from build123d import *

# Parameters (mm, degrees)
SKETCH1_R           = 5
BOSS_EXTRUDE1_DEPTH = 10
CUT_EXTRUDE2_DEPTH  = 10
FILLET1_R           = 2


with BuildPart() as part:
    # Sketch1 → Boss-Extrude1 (new body)
    # profile 1 of 2: a face of its own
    with BuildSketch(Plane.XY):
        with BuildLine():
            Line((0, 0), (0, 100))
            ThreePointArc((0, 100), (25, 125), (50, 100))
            Line((50, 100), (50, 0))
            ThreePointArc((50, 0), (25, -25), (0, 0))
        make_face()
        with BuildLine():
            ThreePointArc((15, 0), (25, -10), (35, 0))
            Line((35, 0), (35, 100))
            ThreePointArc((35, 100), (25, 110), (15, 100))
            Line((15, 100), (15, 0))
        make_face(mode=Mode.SUBTRACT)
    # profile 2 of 2: a face of its own
    with BuildSketch(Plane.XY):
        with BuildLine():
            Line((15, 0), (15, 100))
            ThreePointArc((15, 100), (25, 110), (35, 100))
            Line((35, 100), (35, 0))
            ThreePointArc((35, 0), (25, -10), (15, 0))
        make_face()
        with Locations((25, 0)):
            Circle(SKETCH1_R, mode=Mode.SUBTRACT)
        with Locations((25, 100)):
            Circle(SKETCH1_R, mode=Mode.SUBTRACT)
    extrude(amount=BOSS_EXTRUDE1_DEPTH)

    # Sketch2 → Cut-Extrude2 (cut)
    with BuildSketch(Plane.XY.offset(10)):
        with BuildLine():
            Line((25.064971157, 89.343145751), (10, 89.343145751))
            Line((10, 89.343145751), (10, 70.656854249))
            Line((10, 70.656854249), (26.125631329, 86.782485579))
            ThreePointArc((26.125631329, 86.782485579), (26.450790456, 88.417170899), (25.064971157, 89.343145751))
        make_face()
        with BuildLine():
            Line((40, 69), (40, 89.343145751))
            Line((40, 89.343145751), (22.217514421, 71.560660172))
            ThreePointArc((22.217514421, 71.560660172), (21.892355294, 69.925974851), (23.278174593, 69))
            Line((23.278174593, 69), (40, 69))
        make_face()
        with BuildLine():
            Line((26.721825407, 61), (10, 61))
            Line((10, 61), (10, 40.65685425))
            Line((10, 40.65685425), (22.171572875, 52.828427125))
            Line((22.171572875, 52.828427125), (27.782485579, 58.439339828))
            ThreePointArc((27.782485579, 58.439339828), (28.107644706, 60.074025149), (26.721825407, 61))
        make_face()
        with BuildLine():
            Line((40, 39), (40, 59.343145751))
            Line((40, 59.343145751), (27.828427125, 47.171572875))
            Line((27.828427125, 47.171572875), (22.217514421, 41.560660172))
            ThreePointArc((22.217514421, 41.560660172), (21.892355294, 39.925974852), (23.278174593, 39))
            Line((23.278174593, 39), (40, 39))
        make_face()
        with BuildLine():
            Line((26.721825408, 31.000000001), (10, 31.000000001))
            Line((10, 31.000000001), (10, 10.656854249))
            Line((10, 10.656854249), (27.782485579, 28.439339829))
            ThreePointArc((27.782485579, 28.439339829), (28.107644706, 30.074025149), (26.721825408, 31.000000001))
        make_face()
        with BuildLine():
            Line((40, 9), (40, 29.34314575))
            Line((40, 29.34314575), (22.217514422, 11.560660171))
            ThreePointArc((22.217514422, 11.560660171), (21.892355295, 9.925974851), (23.278174594, 9))
            Line((23.278174594, 9), (40, 9))
        make_face()
    extrude(amount=-CUT_EXTRUDE2_DEPTH, mode=Mode.SUBTRACT)

    # Fillet1
    fillet1_edges = [part.edges().sort_by_distance(p)[0] for p in [
        (10, 10.656854249, 5),
        (10, 31.000000001, 5),
        (40, 59.343145751, 5),
        (40, 39, 5),
        (10, 40.65685425, 5),
        (10, 61, 5),
        (40, 89.343145751, 5),
        (40, 69, 5),
        (40, 29.34314575, 5),
        (40, 9, 5),
        (10, 70.656854249, 5),
        (10, 89.343145751, 5),
    ]]
    fillet(fillet1_edges, radius=FILLET1_R)


solid = part.part
Here's how the part is built. I have some questions about the finished solid (model axes, mm). A direction names the side the tool comes from. Give positions to 0.01 mm unless a question says otherwise; leave off trailing zeros. Write each loop counter-clockwise with the first axis right and the second up, starting at its lowest first coordinate (ties: lowest second). Pieces come first, ordered by that corner, then holes. Notation, with made-up numbers: (82.5, 68) -> (117.5, 68) arc R26 cw to (117.5, 97) -> close; hole circle Ø6 at (38.25, 55). An arc over 180 degrees is marked (long way). Use one line per item in the form item = value. Start each with the question number.
1. Imagine slicing it at B-B on y = -3.5. List the corners of the cut face in (x, z) for me, plus the area to 3 significant figures.
2. Will these pins go through, and if not, where does the flat tip stop? pin 1 Ø2 at (x, z) = (43, 9) entering from +Y; pin 2 Ø5 at (x, z) = (33, 5.5) entering from +Y; pin 3 Ø6 at (x, y) = (25, 0) entering from +Z; pin 4 Ø3 at (x, z) = (19, 5.5) entering from -Y.
3. Imagine slicing it at D-D on x = 42. List the corners of the cut face in (y, z) for me, plus the area to 3 significant figures.
4. Imagine slicing it at C-C on z = 7.75. State how many separate pieces and enclosed holes the cut face has, plus the area to 3 significant figures.
5. On a 3-axis mill with a long thin cutter (end or side, diameter ignored), from which of +Z, -Z, +X, -X, +Y, -Y can I reach the whole of each face in a straight line? I mean faces 3 (the face through (28.117, 60.051, 5.07)), 4 (the face through (25, 51, 10)). Say none if no direction works.
6. If I drill on L1, parallel to X at y = 47, z = 9.25; L2, parallel to X at y = 20, z = 9.5; L3, parallel to Y at x = 35, z = 8.25, over which ranges is the centre line in solid material (lowest first)?
7. Thinking about a two-plate mould opening in Y: for faces 1 (the face through (25, 51, 0)), 2 (the face through (26.46, 88.39, 5.07)), which applies, +Y half, -Y half, draft (parallel to the pull), parting line (faces both ways), or undercut?
8. Imagine slicing it at A-A on x = 17.5. List the corners of the cut face in (y, z) for me, plus the area to 3 significant figures.
Entries:
q1.outline = (0.25, 0) -> (21.43, 0) -> (21.43, 10) -> (0.25, 10) -> close; (28.57, 0) -> (49.75, 0) -> (49.75, 10) -> (28.57, 10) -> close
q1.area = 424 mm²
q2.pin_1 = 118.33
q2.pin_2 = 124.39
q2.pin_3 = through
q2.pin_4 = -24.59
q3.outline = (-18.33, 0) -> (118.33, 0) -> (118.33, 10) -> (-18.33, 10) -> close
q3.area = 1,370 mm²
q4.separate_pieces = 1
q4.enclosed_holes = 8
q4.area = 5,650 mm²
q5.face_3 = +Z, -Z
q5.face_4 = +Z, +X, -X, +Y, -Y
q6.L1 = 0 to 10, 16.34 to 27.66, 40 to 50
q6.L2 = 0 to 10, 19.34 to 30.66, 40 to 50
q6.L3 = -22.91 to 9, 24.34 to 39, 54.34 to 69, 84.34 to 122.91
q7.face_1 = draft
q7.face_2 = undercut
q8.outline = (-23.85, 0) -> (18.16, 0) -> (18.16, 10) -> (-23.85, 10) -> close; (31, 0) -> (48.16, 0) -> (48.16, 10) -> (31, 10) -> close; (61, 0) -> (78.16, 0) -> (78.16, 10) -> (61, 10) -> close; (89.34, 0) -> (123.85, 0) -> (123.85, 10) -> (89.34, 10) -> close
q8.area = 1,110 mm²
